from build123d import *

# Parameters (mm, degrees)
SKETCH1_R           = 4
BOSS_EXTRUDE1_DEPTH = 26
SKETCH2_R           = 6.5
BOSS_EXTRUDE2_DEPTH = 4
CUT_EXTRUDE1_START  = -18
SKETCH3_R           = 4
SKETCH3_R_2         = 3.7
CUT_EXTRUDE1_DEPTH  = 18
FILLET2_R           = 2
CHAMFER1_SIZE       = 2
CHAMFER1_SIZE2      = 1.154700538
FILLET3_R           = 1


with BuildPart() as part:
    # Sketch1 → Boss-Extrude1 (new body)
    with BuildSketch(Plane(origin=(0, 0, 0), x_dir=(1, 0, 0), z_dir=(0, 1, 0))):
        with Locations(Location((0, 0, 0), (0, 0, 90))):
            Circle(SKETCH1_R)
    extrude(amount=BOSS_EXTRUDE1_DEPTH)

    # Sketch2 → Boss-Extrude2 (add)
    with BuildSketch(Plane.XZ):
        with Locations(Location((0, 0, 0), (0, 0, 270))):
            Circle(SKETCH2_R)
    extrude(amount=BOSS_EXTRUDE2_DEPTH)

    # Sketch3 → Cut-Extrude1 (cut)
    with BuildSketch(Plane(origin=(0, 26, 0), x_dir=(1, 0, 0), z_dir=(0, 1, 0)).offset(CUT_EXTRUDE1_START)):
        with Locations(Location((0, 0, 0), (0, 0, 90))):
            Circle(SKETCH3_R)
        with Locations(Location((0, 0, 0), (0, 0, 270))):
            Circle(SKETCH3_R_2, mode=Mode.SUBTRACT)
    extrude(amount=CUT_EXTRUDE1_DEPTH, mode=Mode.SUBTRACT)

    # Fillet2
    fillet2_edges = [part.edges().sort_by_distance(p)[0] for p in [
        (0, -4, 6.5),
    ]]
    fillet(fillet2_edges, radius=FILLET2_R)

    # Chamfer1
    chamfer1_edges = [part.edges().sort_by_distance(p)[0] for p in [
        (0, 26, -3.7),
    ]]
    chamfer1_side = [part.faces().sort_by_distance(p)[0] for p in [
        (0, 17, -3.7),
    ]]
    chamfer(chamfer1_edges, length=CHAMFER1_SIZE, length2=CHAMFER1_SIZE2, reference=chamfer1_side[0])

    # Fillet3
    fillet3_edges = [part.edges().sort_by_distance(p)[0] for p in [
        (0, 26, -2.545299462),
        (0, 24, -3.7),
    ]]
    fillet(fillet3_edges, radius=FILLET3_R)


solid = part.part
Work out the finished part from the listing and answer in its coordinate system (mm). A direction names the side the tool comes from. Give positions to 0.01 mm unless a question says otherwise; leave off trailing zeros. Order: outer loops, then holes, each group sorted by start corner. A loop starts at its lowest first (then second) coordinate and runs counter-clockwise, first axis right, second up. Notation, with made-up numbers: (7.25, -9.75) -> (56.25, -9.75) arc R16 ccw to (56.25, -0.75) -> close; hole circle Ø4 at (-6, 6). An arc over 180 degrees is marked (long way). One line per item, written item: value.
Item 1: Straight lines are drawn through the part: probe 1 along Y at (x, z) = (-3.75, 1); probe 2 along Y at (x, z) = (-1, -4); probe 3 along X at (y, z) = (3, 0). For each, find the intervals that lie inside material, in ascending order.
Answer sheet:
probe 1: -4 to 8
probe 2: -4 to 0
probe 3: -4 to 4
Item 2: Find section B-B, the plane y = 4. Give the vertices of the cut face in (x, z).
Answer sheet:
outline: circle Ø8 at (0, 0)
Item 3: Flat-ended cylindrical pins translate along their axes: P1, Ø5, axis at y = 12.5, z = 2.5, coming from the +X side; P2, Ø1, axis at y = 22.5, z = 2, coming from the +X side. Find the tip coordinate at first contact, or state that the pin passes through.
Answer sheet:
P1: x = 3.7
P2: x = 3.38
Item 4: A tool of negligible diameter and unlimited length cuts with its end or side. For faces 1 (the cylindrical face through (-3.612, 15.756, -0.802)), 2 (the cylindrical face through (-3.955, -0.986, 5.158)), from which of +Z, -Z, +X, -X, +Y, -Y can it reach the whole face along a straight path? Write none if from no direction.
Answer sheet:
face 1: +Y
face 2: +Y, -Y
Item 5: Find section A-A, the plane y = 9.5. Give the vertices of the cut face in (x, z).
Answer sheet:
outline: circle Ø7.4 at (0, 0)
